Could you check a few things on this model? Use its own coordinates, in mm. A direction names the side the tool comes from. Round coordinates to 2 decimals unless told otherwise and drop trailing zeros. Order: outer loops, then holes, each group sorted by start corner. A loop starts at its lowest first (then second) coordinate and runs counter-clockwise, first axis right, second up.
```python
from build123d import *

# Parameters (mm, degrees)
SKETCH1_W           = 12.7
SKETCH1_H           = 12.7
BOSS_EXTRUDE1_DEPTH = 2.54
FILLET1_R           = 0.635
SHELL1_START        = 0.635
SHELL1_OUTLINE_W    = 1.905
SHELL1_OUTLINE_H    = 11.43
SHELL1_DEPTH        = 11.43
SKETCH2_R           = 2.54
BOSS_EXTRUDE2_DEPTH = 1.905
BOSS_EXTRUDE3_DEPTH = 0.00254


# Read off the part's stored shape, not the designer's step: Shell1
with BuildPart() as part:
    # Sketch1 → Boss-Extrude1 (new body)
    with BuildSketch(Plane(origin=(0, 0, 0), x_dir=(1, 0, 0), z_dir=(0, 1, 0))):
        with Locations((6.35, 6.35)):
            Rectangle(SKETCH1_W, SKETCH1_H)
    extrude(amount=BOSS_EXTRUDE1_DEPTH)

    # Fillet1
    fillet1_edges = [part.edges().sort_by_distance(p)[0] for p in [
        (0, 1.27, -12.7),
        (12.7, 1.27, -12.7),
        (12.7, 1.27, 0),
        (0, 1.27, 0),
    ]]
    fillet(fillet1_edges, radius=FILLET1_R)

    # Shell1 outline → Shell1 (cut)
    with BuildSketch(Plane.YZ.offset(SHELL1_START)):
        with Locations((0.9525, -6.35)):
            Rectangle(SHELL1_OUTLINE_W, SHELL1_OUTLINE_H)
    extrude(amount=SHELL1_DEPTH, mode=Mode.SUBTRACT)

    # Sketch2 → Boss-Extrude2 (add)
    with BuildSketch(Plane(origin=(0, 1.905, 0), x_dir=(-1, 0, 0), z_dir=(0, -1, 0))):
        with Locations(Location((-6.35, 6.35, 0), (0, 0, 270))):
            Circle(SKETCH2_R)
    extrude(amount=BOSS_EXTRUDE2_DEPTH)

    # Sketch3 → Boss-Extrude3 (add)
    with BuildSketch(Plane(origin=(0, 2.54, 0), x_dir=(1, 0, 0), z_dir=(0, 1, 0))):
        with BuildLine():
            Line((7.589389744, 5.278208534), (8.128096675, 4.581769231))
            Line((8.128096675, 4.581769231), (7.418937019, 4.581769231))
            Line((7.418937019, 4.581769231), (7.13972528, 4.942391226))
            add(Edge.make_bspline(
                [(7.13972528, 4.942391226), (7.110478697, 4.926466187), (7.052123488, 4.894691228), (6.960614822, 4.855068108), (6.867412166, 4.820307815), (6.771164987, 4.793069664), (6.672797341, 4.771629932), (6.571799543, 4.755260346), (6.468243861, 4.746629027), (6.398354698, 4.745272899), (6.363147756, 4.744589744)],
                knots=[0, 0, 0, 0, 0.985706899, 1.966764212, 2.949968678, 3.929638882, 4.925906056, 5.930211904, 6.957336097, 8, 8, 8, 8], degree=3))
            add(Edge.make_bspline(
                [(6.363147756, 4.744589744), (6.304542849, 4.745905131), (6.189596707, 4.748485098), (6.021255045, 4.773257837), (5.86010189, 4.81065794), (5.706735433, 4.865301405), (5.560639002, 4.93474107), (5.422980515, 5.020794933), (5.292158769, 5.121077116), (5.171374474, 5.236571809), (5.060858729, 5.361731796), (4.96429439, 5.49470483), (4.88220836, 5.633416247), (4.815264882, 5.778083639), (4.763209523, 5.928956411), (4.726755567, 6.085622481), (4.703644343, 6.248298361), (4.700779646, 6.358724268), (4.699325641, 6.414772035)],
                knots=[0, 0, 0, 0, 1.070144486, 2.098953612, 3.10240755, 4.088674545, 5.067611437, 6.052256776, 7.0494179, 8.074208254, 9.100739571, 10.09639475, 11.072322686, 12.041159829, 13.004031207, 13.983083054, 14.976293755, 16, 16, 16, 16], degree=3))
            add(Edge.make_bspline(
                [(4.699325641, 6.414772035), (4.69981035, 6.452327381), (4.700773631, 6.526962536), (4.712359176, 6.637570612), (4.729074707, 6.74600964), (4.753617357, 6.851696745), (4.783880127, 6.95540729), (4.822385353, 7.056316673), (4.867009306, 7.15538311), (4.918202859, 7.251783598), (4.976351833, 7.344092805), (5.03814397, 7.433044208), (5.106877934, 7.51578176), (5.18012093, 7.594168735), (5.258113534, 7.668153791), (5.342084012, 7.736211938), (5.430436693, 7.800032133), (5.523808175, 7.858276403), (5.6205775, 7.910923569), (5.719854021, 7.956677527), (5.820882117, 7.995819583), (5.923699482, 8.027705354), (6.028618864, 8.051600525), (6.134717058, 8.0697941), (6.242956128, 8.079914479), (6.315639078, 8.081572932), (6.352335457, 8.082410256)],
                knots=[0, 0, 0, 0, 1.035855852, 2.058595393, 3.065553363, 4.06176554, 5.050183643, 6.044349766, 7.039272903, 8.046842428, 9.053256483, 10.04817962, 11.033146707, 12.018200652, 13.007259073, 13.996749908, 14.99846043, 16.012935138, 17.03119782, 18.036301871, 19.027088812, 20.018894167, 21.003704893, 21.994284571, 22.987348552, 24, 24, 24, 24], degree=3))
            add(Edge.make_bspline(
                [(6.352335457, 8.082410256), (6.407752886, 8.081001093), (6.516953024, 8.078224334), (6.677585719, 8.054480547), (6.832490656, 8.016657267), (6.981029087, 7.962010037), (7.12410888, 7.893107178), (7.260304055, 7.807850891), (7.391055808, 7.707999288), (7.513539447, 7.593504419), (7.626732359, 7.469249914), (7.725409869, 7.33593868), (7.808946318, 7.196116061), (7.878612035, 7.049726313), (7.931097461, 6.895913898), (7.968565757, 6.735700032), (7.992282098, 6.568971999), (7.995039629, 6.455345392), (7.996441026, 6.397599559)],
                knots=[0, 0, 0, 0, 1.015551519, 2.00114601, 2.970254478, 3.93428303, 4.897362978, 5.876714212, 6.874912676, 7.909046156, 8.946527051, 9.952474942, 10.9443724, 11.928494229, 12.919233427, 13.917651329, 14.941735923, 16, 16, 16, 16], degree=3))
            add(Edge.make_bspline(
                [(7.996441026, 6.397599559), (7.995275963, 6.344324576), (7.992984514, 6.239543185), (7.973133051, 6.085073676), (7.941799009, 5.93618576), (7.89679568, 5.792773627), (7.839764108, 5.654993593), (7.768702598, 5.523255836), (7.686759711, 5.39599636), (7.622008209, 5.317666883), (7.589389744, 5.278208534)],
                knots=[0, 0, 0, 0, 1.049646143, 2.064447078, 3.064298101, 4.044929938, 5.022708814, 5.998521441, 6.991758374, 8, 8, 8, 8], degree=3))
        make_face()
        with BuildLine():
            add(Edge.make_bspline(
                [(7.215411378, 5.762853966), (7.232374671, 5.787174078), (7.265910436, 5.835253985), (7.308344006, 5.911515257), (7.344794922, 5.989262448), (7.374938402, 6.068903528), (7.397868514, 6.150894907), (7.414166719, 6.234701319), (7.424959684, 6.320361144), (7.42602991, 6.378062342), (7.426569231, 6.407139824)],
                knots=[0, 0, 0, 0, 1.031533623, 2.039301536, 3.033003023, 4.018477747, 4.999688364, 5.992485227, 6.988348989, 8, 8, 8, 8], degree=3))
            add(Edge.make_bspline(
                [(7.426569231, 6.407139824), (7.425565467, 6.44492283), (7.423589712, 6.519292914), (7.408750209, 6.628618034), (7.383890189, 6.733390986), (7.349226622, 6.833868214), (7.305573348, 6.930307641), (7.250735612, 7.021906242), (7.186308475, 7.109139766), (7.112913869, 7.191168117), (7.03300641, 7.266242217), (6.948022887, 7.332360438), (6.858546258, 7.388140444), (6.764524178, 7.433179158), (6.666976563, 7.469454645), (6.564856578, 7.493802938), (6.459054311, 7.50976733), (6.386951725, 7.511606706), (6.350427404, 7.512538462)],
                knots=[0, 0, 0, 0, 1.056263418, 2.079093448, 3.078410197, 4.062632158, 5.04680056, 6.032966551, 7.041959893, 8.074807684, 9.106532056, 10.103754224, 11.080880922, 12.048629763, 13.014470275, 13.984975, 14.979267944, 16, 16, 16, 16], degree=3))
            add(Edge.make_bspline(
                [(6.350427404, 7.512538462), (6.312851373, 7.511555352), (6.238893703, 7.509620382), (6.130317465, 7.494494694), (6.026169919, 7.470769489), (5.926998511, 7.435934883), (5.832502968, 7.392042518), (5.742687623, 7.338185734), (5.658002596, 7.274062961), (5.578246545, 7.201552409), (5.506184165, 7.121091877), (5.442548821, 7.034811209), (5.38928769, 6.942918458), (5.344683443, 6.846250439), (5.311105764, 6.743724644), (5.287189539, 6.636142959), (5.272075339, 6.523320349), (5.270170179, 6.446409309), (5.269197436, 6.407139824)],
                knots=[0, 0, 0, 0, 1.042613217, 2.052085894, 3.036973397, 4.002832266, 4.963730975, 5.924467509, 6.903642813, 7.907474205, 8.911719447, 9.896835452, 10.877830278, 11.85475743, 12.846581833, 13.865885605, 14.910357018, 16, 16, 16, 16], degree=3))
            add(Edge.make_bspline(
                [(5.269197436, 6.407139824), (5.270486861, 6.363620201), (5.273013922, 6.278328951), (5.290802543, 6.153911765), (5.321215888, 6.036399284), (5.365204909, 5.926425933), (5.419563509, 5.822443324), (5.488046054, 5.726666097), (5.567678666, 5.637200516), (5.629149275, 5.585123602), (5.660348277, 5.558692308)],
                knots=[0, 0, 0, 0, 1.078047314, 2.112794111, 3.106520711, 4.077995885, 5.041371964, 6.006121678, 6.988020189, 8, 8, 8, 8], degree=3))
            add(Edge.make_bspline(
                [(5.660348277, 5.558692308), (5.685874998, 5.539126434), (5.73649664, 5.500325655), (5.817588059, 5.451211693), (5.900701996, 5.408546176), (5.986624335, 5.374435559), (6.075058256, 5.347307518), (6.165984953, 5.328515818), (6.259582038, 5.316554097), (6.32282995, 5.315165288), (6.354879527, 5.314461538)],
                knots=[0, 0, 0, 0, 1.027457745, 2.037535419, 3.025615023, 4.011018129, 4.9886297, 5.978868484, 6.975833209, 8, 8, 8, 8], degree=3))
            add(Edge.make_bspline(
                [(6.354879527, 5.314461538), (6.391651355, 5.315632394), (6.464636665, 5.317956327), (6.57206456, 5.338199851), (6.676734184, 5.368474506), (6.742353753, 5.399420844), (6.775287179, 5.414952324)],
                knots=[0, 0, 0, 0, 1.010952568, 2.006554787, 2.999521277, 4, 4, 4, 4], degree=3))
            Line((6.775287179, 5.414952324), (6.223859896, 6.128564103))
            Line((6.223859896, 6.128564103), (6.933019551, 6.128564103))
            Line((6.933019551, 6.128564103), (7.215411378, 5.762853966))
        make_face(mode=Mode.SUBTRACT)
    extrude(amount=BOSS_EXTRUDE3_DEPTH)


solid = part.part
```
Q1. We'd pull the mould along Z, two halves only. Please class faces 3 (the flat face through (6, 1, -0.635)), 4 (the flat face through (5, 2.54, -8)), 5 (the flat face through (5, 1.905, -9)), 6 (the flat face through (6, 1, -12.7)): released by +Z, released by -Z, zero draft, split by the parting line, or undercut.
Q2. For faces 1 (the flat face through (12.065, 1, -6)), 2 (the flat face through (6, 1, 0)), which set-ups out of +Z, -Z, +X, -X, +Y, -Y let a thin tool reach every point of the face, with its end or its side?
Q3. For P1, Ø1.5, axis at x = 5, z = -2, coming from the +Y side, with a flat end and sliding along its axis, tell me the tip position at first contact or that it passes through.
Q4. Imagine slicing it at A-A, the plane y = 0.35. Please give me the cut outline in (x, z) (3 decimals), then the cut area to 3 significant figures.
Q5. Imagine slicing it at D-D, the plane x = 8.5. Please give me the cut outline in (y, z) (3 decimals), then the cut area to 3 significant figures.
Q6. I need wall thicknesses on L1, parallel to X at y = 1.2, z = -7.75 (3 decimals); L2, parallel to Z at x = 4.5, y = 1.75 (3 decimals); L3, parallel to Z at x = 8.5, y = 1 (3 decimals). Which ranges of each line are inside material? Lowest first, please.
Q7. Imagine slicing it at C-C, the plane z = -9.25. Please give me the cut outline in (x, y) (3 decimals), then the cut area to 3 significant figures.
Q8. Imagine slicing it at B-B, the plane x = 1. Please give me the cut outline in (y, z) (3 decimals), then the cut area to 3 significant figures.
Filled in:
1. face 3: undercut
1. face 4: zero draft
1. face 5: undercut
1. face 6: released by -Z
2. face 1: -Y
2. face 2: +Z, +X, -X, +Y, -Y
3. P1: stops at y = 2.54
4. outline: (0, -12.065) arc R0.635 ccw to (0.635, -12.7) - (12.065, -12.7) arc R0.635 ccw to (12.7, -12.065) - (12.7, -0.635) arc R0.635 ccw to (12.065, 0) - (0.635, 0) arc R0.635 ccw to (0, -0.635) - close; circle Ø5.08 at (6.35, -6.35); hole (0.635, -12.065) - (12.065, -12.065) - (12.065, -0.635) - (0.635, -0.635) - close
4. area: 50.6 mm2
5. outline: (0, -12.7) - (2.54, -12.7) - (2.54, 0) - (0, 0) - (0, -0.635) - (1.905, -0.635) - (1.905, -4.998) - (0, -4.998) - (0, -7.702) - (1.905, -7.702) - (1.905, -12.065) - (0, -12.065) - close
5. area: 15.6 mm2
6. L1: x = 0 to 0.635, 4.231 to 8.469, 12.065 to 12.7
6. L2: z = -12.7 to -12.065, -8.09 to -4.61, -0.635 to 0
6. L3: z = -12.7 to -12.065, -7.702 to -4.998, -0.635 to 0
7. outline: (0, 0) - (0.635, 0) - (0.635, 1.905) - (12.065, 1.905) - (12.065, 0) - (12.7, 0) - (12.7, 2.54) - (0, 2.54) - close
7. area: 10.5 mm2
8. outline: (0, -12.7) - (2.54, -12.7) - (2.54, 0) - (0, 0) - (0, -0.635) - (1.905, -0.635) - (1.905, -12.065) - (0, -12.065) - close
8. area: 10.5 mm2
